Autodesk Inventor part; units mm, degrees
ref_plane "YZ Plane" through (0, 0, 0) normal (1, 0, 0) x (0, 1, 0)
ref_plane "XZ Plane" through (0, 0, 0) normal (0, 1, 0) x (-1, 0, 0)
ref_plane "XY Plane" through (0, 0, 0) normal (0, 0, 1) x (1, 0, 0)
sketch "Sketch1" plane through (0, 0, 0) normal (0, 0, 1) x (1, 0, 0)
  line L0 (-15, 15) -> (15, 15)
  line L1 (15, 15) -> (15, -15)
  line L2 (15, -15) -> (-15, -15)
  line L3 (-15, -15) -> (-15, 15)
  point P0 (0, 0)
  point P1 (0, 15)
  point P2 (-15, 0)
  dimension "d0" = 30
  dimension "d1" = 30
extrude "Extrusion1" add sketch "Sketch1" along normal blind 30
sketch "Sketch6" plane through (15, -15, 0) normal (1, 0, 0) x (0, 0, -1)
  circle A0 centre (-25, 5) radius 2.25
  circle A1 centre (-25, 25) radius 2.25
  line L0 (-30, 0) -> (-30, 30)
  line L1 (0, 0) -> (-30, 0)
  line L2 (0, 30) -> (-30, 30)
  point P0 (0, 15)
  dimension "d19" = 4.5
  dimension "d20" = 5
  dimension "d21" = 5
  dimension "d22" = 5
extrude "Extrusion4" cut sketch "Sketch6" against normal through all
sketch "Sketch4" plane through (0, 0, 0) normal (0, 0, -1) x (-1, 0, 0)
  line L0 (2, -15) -> (-8, -15)
  line L1 (-8, -15) -> (-8, 15)
  line L2 (-8, 15) -> (2, 15)
  line L3 (2, 15) -> (2, -15)
  line L4 (15, -15) -> (-15, -15)
  line L5 (-15, 15) -> (15, 15)
  line L6 (-15, -15) -> (-15, 15)
  point P0 (0, 0)
  dimension "d8" = 10
  dimension "d25" = 7
extrude "Extrusion3" cut sketch "Sketch4" against normal blind 15 contours L0 L1 L2 L3
sketch "Sketch5" plane through (15, -15, 0) normal (1, 0, 0) x (0, 0, -1)
  line L0 (0, 0) -> (0, 30)
  point P0 (0, 15)
  point P1 (-5, 15)
  point P2 (0, 15)
  dimension "d11" = 5
hole "Hole1" at (15, 0, 5) direction (-1, 0, 0) diameter 5 depth 10 tip angle 118
sketch "Sketch7" plane through (-2, -15, 0) normal (1, 0, 0) x (0, 0, -1)
  circle A0 centre (-5, 15) radius 2.5
  point P0 (0, 15)
hole "Hole2" at (-2, 0, 5) direction (-1, 0, 0) diameter 4.134 end through all
equation "\"d22\" = d21"
properties part number "0005-10-018 intinzator x" material "Wood (Maple)"
Model file for the job. Use its own axes, mm. A direction names the side the tool comes from. Give positions to 0.01 mm unless a question says otherwise; leave off trailing zeros. Order: outer loops, then holes, each group sorted by start corner. A loop starts at its lowest first (then second) coordinate and runs counter-clockwise, first axis right, second up. Notation, with made-up numbers: (4, 41) - (16, 41) arc R18 cw to (16, 63) - close; hole circle Ø5 at (28, -9.5). An arc over 180 degrees is marked (long way). One line per item, written item: value.
Item 1: Wall check: line 1 (Y direction, x = 0.5, z = 25); line 2 (Y direction, x = -5, z = 5); line 3 (Y direction, x = -11.75, z = 23.75). Give the ranges that are in metal, low to high.
Response values:
line 1: -15 to -12.25, -7.75 to 7.75, 12.25 to 15
line 2: -15 to -2.07, 2.07 to 15
line 3: -15 to -11.87, -8.13 to 8.13, 11.87 to 15
Item 2: Slice it at C-C (y = -10). List the corners of the cut face in (x, z).
Response values:
outline: (-15, 0) - (-2, 0) - (-2, 15) - (8, 15) - (8, 0) - (15, 0) - (15, 22.75) - (-15, 22.75) - close; (-15, 27.25) - (15, 27.25) - (15, 30) - (-15, 30) - close
Item 3: Tool access for faces 1 (the cylindrical face through (11.451, -0.751, 2.615)), 2 (the cylindrical face through (0.21, 10.676, 22.854)), 3 (the flat face through (8, 0, 9)): list every direction of +Z, -Z, +X, -X, +Y, -Y with a clear straight run to the whole face (end or side of a thin tool).
Response values:
face 1: +X
face 2: +X, -X
face 3: -Z, +Y, -Y
Item 4: Slice it at D-D (z = 5). List the corners of the cut face in (x, y).
Response values:
outline: (-15, -15) - (-2, -15) - (-2, -2.07) - (-15, -2.07) - close; (-15, 2.07) - (-2, 2.07) - (-2, 15) - (-15, 15) - close; (8, -15) - (15, -15) - (15, -2.5) - (8, -2.5) - close; (8, 2.5) - (15, 2.5) - (15, 15) - (8, 15) - close
Item 5: Two-plate mould, pull along Y, no slides. Class faces 4 (the cylindrical face through (0.21, -8.103, 23.79)), 5 (the flat face through (11, 0, 0)), 6 (the flat face through (0, 15, 18)): released by +Y, released by -Y, zero draft, split by the parting line, or undercut.
Response values:
face 4: undercut
face 5: zero draft
face 6: released by +Y
Item 6: Slice it at A-A (x = -5). List the corners of the cut face in (y, z).
Response values:
outline: (-15, 0) - (15, 0) - (15, 30) - (-15, 30) - close; hole circle Ø4.5 at (-10, 25); hole circle Ø4.13 at (0, 5); hole circle Ø4.5 at (10, 25)
Item 7: Slice it at B-B (z = 13.25). List the corners of the cut face in (x, y).
Response values:
outline: (-15, -15) - (-2, -15) - (-2, 15) - (-15, 15) - close; (8, -15) - (15, -15) - (15, 15) - (8, 15) - close
